Geometry check sheet. Reference: the model listing, model coordinates, mm. A direction names the side the tool comes from. Give positions to 0.01 mm unless a question says otherwise; leave off trailing zeros. Order: outer loops, then holes, each group sorted by start corner. A loop starts at its lowest first (then second) coordinate and runs counter-clockwise, first axis right, second up. Notation, with made-up numbers: M 85.25,-7 L 139.25,-7 A21 ccw 139.25,6 Z; hole C -5.75,42.25 d3. An arc over 180 degrees is marked long. Answer as CSV lines item,"result".
from build123d import *

# Parameters (mm, degrees)
SKETCH1_W            = 43.7
SKETCH1_H            = 60.2
SKETCH1_R            = 1.7
SKETCH1_R_2          = 10.2
BOSS_EXTRUDE2_DEPTH  = 8
SKETCH7_W            = 20
SKETCH7_H            = 3
BOSS_EXTRUDE7_DEPTH  = 10
SKETCH8_W            = 20
SKETCH8_H            = 3
BOSS_EXTRUDE8_DEPTH  = 3
SKETCH9_W            = 20
SKETCH9_H            = 3
BOSS_EXTRUDE9_DEPTH  = 10
SKETCH10_W           = 20
SKETCH10_H           = 3.203201764
BOSS_EXTRUDE10_DEPTH = 10


with BuildPart() as part:
    # Sketch1 → Boss-Extrude2 (new body)
    with BuildSketch(Plane(origin=(0, 0, 0), x_dir=(1, 0, 0), z_dir=(0, 1, 0))):
        with Locations((-1.85, 30.1)):
            Rectangle(SKETCH1_W, SKETCH1_H)
        with Locations(Location((7, 27.375644347, 0), (0, 0, 270))):
            Circle(SKETCH1_R, mode=Mode.SUBTRACT)
        with Locations(Location((7.5, 52.490381057, 0), (0, 0, 270))):
            Circle(SKETCH1_R, mode=Mode.SUBTRACT)
        with Locations(Location((0, 53.5, 0), (0, 0, 270))):
            Circle(SKETCH1_R, mode=Mode.SUBTRACT)
        with Locations(Location((-15, 39.5, 0), (0, 0, 270))):
            Circle(SKETCH1_R, mode=Mode.SUBTRACT)
        with Locations(Location((12.124355653, 32.5, 0), (0, 0, 270))):
            Circle(SKETCH1_R, mode=Mode.SUBTRACT)
        with Locations(Location((0, 39.5, 0), (0, 0, 270))):
            Circle(SKETCH1_R_2, mode=Mode.SUBTRACT)
        with Locations(Location((-12.124355653, 32.5, 0), (0, 0, 270))):
            Circle(SKETCH1_R, mode=Mode.SUBTRACT)
    extrude(amount=BOSS_EXTRUDE2_DEPTH)

    # Sketch7 → Boss-Extrude7 (add)
    with BuildSketch(Plane.XZ):
        with Locations((10, -1.5)):
            Rectangle(SKETCH7_W, SKETCH7_H)
    extrude(amount=BOSS_EXTRUDE7_DEPTH)

    # Sketch8 → Boss-Extrude8 (add)
    with BuildSketch(Plane(origin=(0, 8, 0), x_dir=(1, 0, 0), z_dir=(0, 1, 0))):
        with Locations((10, 1.5)):
            Rectangle(SKETCH8_W, SKETCH8_H)
    extrude(amount=BOSS_EXTRUDE8_DEPTH)

    # Sketch9 → Boss-Extrude9 (add)
    with BuildSketch(Plane.XY):
        with Locations((10, 9.5)):
            Rectangle(SKETCH9_W, SKETCH9_H)
    extrude(amount=BOSS_EXTRUDE9_DEPTH)

    # Sketch10 → Boss-Extrude10 (add)
    with BuildSketch(Plane(origin=(0, 11, 0), x_dir=(1, 0, 0), z_dir=(0, 1, 0))):
        with Locations((10, -8.398399118)):
            Rectangle(SKETCH10_W, SKETCH10_H)
    extrude(amount=BOSS_EXTRUDE10_DEPTH)


solid = part.part
(1) Section check B-B on x = -15. Enter the section's corners in (y, z), then the cut area to 3 significant figures.
The answers:
outline,"M 0,-60.2 L 8,-60.2 L 8,-41.2 L 0,-41.2 Z; M 0,-37.8 L 8,-37.8 L 8,0 L 0,0 Z"
area,"454 mm2"
(2) Draft check along X on faces 1 (the face through (0.07, 3.94, -55.2)), 2 (the face through (10, -10, -1)), 3 (the face through (0, -5, -2)). Enter one of: +X half, -X half, draft (parallel to the pull), parting line (faces both ways), or undercut.
The answers:
face 1,"undercut"
face 2,"draft"
face 3,"-X half"
(3) Section check A-A on z = -39.5. Enter the section's corners in (x, y).
The answers:
outline,"M -23.7,0 L -16.7,0 L -16.7,8 L -23.7,8 Z; M -13.3,0 L -10.2,0 L -10.2,8 L -13.3,8 Z; M 10.2,0 L 20,0 L 20,8 L 10.2,8 Z"
(4) Section check D-D on z = -21. Enter the section's corners in (x, y), then the cut area to 3 significant figures.
The answers:
outline,"M -23.7,0 L 20,0 L 20,8 L -23.7,8 Z"
area,"350 mm2"
(5) Gauge pin test, flat ends, axial feed: P1, Ø5.5, axis at x = -15, z = -39.5, coming from the -Y side; P2, Ø3, axis at x = 12.5, z = 4, coming from the +Y side; P3, Ø9, axis at x = -2, y = -4.5, coming from the +Z side; P4, Ø2, axis at x = 12.12, z = -32.5, coming from the +Y side. Record the tip position at first contact, or that the pin passes through.
The answers:
P1,"stops at y = 0"
P2,"stops at y = 11"
P3,"stops at z = 0"
P4,"passes through"
(6) Section check C-C on y = 18.5. Enter the section's corners in (x, z).
The answers:
outline,"M 0,6.8 L 20,6.8 L 20,10 L 0,10 Z"
(7) Tool access check on faces 4 (the face through (0, 12, 8)), 5 (the face through (6.89, 3.94, -47.02)), 6 (the face through (3, 1, 0)), 7 (the face through (10, -5, -3)), 8 (the face through (10, 11, 2)). Record the directions out of +Z, -Z, +X, -X, +Y, -Y that give a thin tool (end or side, any length) a straight path to the whole face; none if there is none.
The answers:
face 4,"+Z, -Z, -X, +Y"
face 5,"+Y, -Y"
face 6,"+Z, +X, -X, -Y"
face 7,"-Z, +X, -X, -Y"
face 8,"-Z, +X, -X, +Y"
(8) Material ranges on line 1 (X direction, y = 2.5, z = -39.5); line 2 (X direction, y = 3, z = -53); line 3 (Y direction, x = -13.5, z = -38.5), recorded low to high.
The answers:
line 1,"x = -23.7 to -16.7, -13.3 to -10.2, 10.2 to 20"
line 2,"x = -23.7 to -1.62, 1.62 to 5.88, 9.12 to 20"
line 3,"y = 0 to 8"
